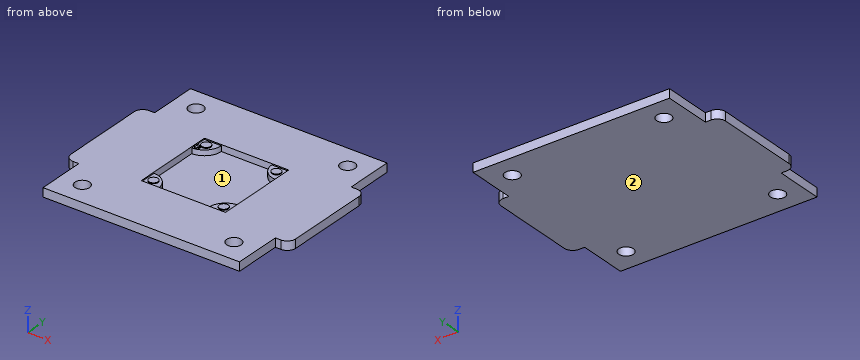
from build123d import *

# Parameters (mm, degrees)
SKETCH_1_W          = 70
SKETCH_1_H          = 70
EXTRUDE_1_DEPTH     = 3.1
SKETCH_2_W          = 30
SKETCH_2_H          = 30
CUT_EXTRUDE_1_DEPTH = 2.3
SKETCH_3_R          = 2.6
CUT_EXTRUDE_2_DEPTH = 4.1
EXTRUDE_2_DEPTH     = 2.7
SKETCH_6_R          = 1.6
EXTRUDE_3_DEPTH     = 0.3


with BuildPart() as part:
    # 草图1 → 凸台-拉伸1 (new body)
    with BuildSketch(Plane.XY):
        with BuildLine():
            Line((-2, 17), (0, 17))
            Line((0, 17), (0, 53))
            Line((0, 53), (-2, 53))
            ThreePointArc((-2, 53), (-4.121320344, 52.121320344), (-5, 50))
            Line((-5, 50), (-5, 20))
            ThreePointArc((-5, 20), (-4.121320344, 17.878679656), (-2, 17))
        make_face()
        with Locations((35, 35)):
            Rectangle(SKETCH_1_W, SKETCH_1_H)
        with BuildLine():
            Line((70, 53), (70, 17))
            Line((70, 17), (72, 17))
            ThreePointArc((72, 17), (74.121320344, 17.878679656), (75, 20))
            Line((75, 20), (75, 50))
            ThreePointArc((75, 50), (74.121320344, 52.121320344), (72, 53))
            Line((72, 53), (70, 53))
        make_face()
    extrude(amount=EXTRUDE_1_DEPTH)

    # 草图2 → 切除-拉伸1 (cut)
    with BuildSketch(Plane.XY.offset(3.1)):
        with Locations((35, 35)):
            Rectangle(SKETCH_2_W, SKETCH_2_H)
    extrude(amount=-CUT_EXTRUDE_1_DEPTH, mode=Mode.SUBTRACT)

    # 草图3 → 切除-拉伸2 (cut, through all)
    with BuildSketch(Plane.XY.offset(3.1)):
        with Locations((8, 62)):
            Circle(SKETCH_3_R)
        with Locations((62, 62)):
            Circle(SKETCH_3_R)
        with Locations((8, 8)):
            Circle(SKETCH_3_R)
        with Locations((62, 8)):
            Circle(SKETCH_3_R)
    extrude(amount=-CUT_EXTRUDE_2_DEPTH, mode=Mode.SUBTRACT)

    # 草图4 → 凸台-拉伸2 (add)
    with BuildSketch(Plane.XY):
        with BuildLine():
            Line((20, 44), (20, 50))
            Line((20, 50), (26, 50))
            ThreePointArc((26, 50), (24.242640687, 45.757359313), (20, 44))
        make_face()
        with BuildLine():
            Line((50, 44), (50, 50))
            Line((50, 50), (44, 50))
            ThreePointArc((44, 50), (45.757359313, 45.757359313), (50, 44))
        make_face()
        with BuildLine():
            Line((50, 20), (44, 20))
            ThreePointArc((44, 20), (45.757359313, 24.242640687), (50, 26))
            Line((50, 26), (50, 20))
        make_face()
        with BuildLine():
            Line((20, 26), (20, 20))
            Line((20, 20), (26, 20))
            ThreePointArc((26, 20), (24.242640687, 24.242640687), (20, 26))
        make_face()
    extrude(amount=EXTRUDE_2_DEPTH)

    # 草图6 → 凸台-拉伸3 (add)
    with BuildSketch(Plane.XY.offset(2.7)):
        with Locations((22.5, 47.5)):
            Circle(SKETCH_6_R)
        with Locations((47.5, 47.5)):
            Circle(SKETCH_6_R)
        with Locations((47.5, 22.5)):
            Circle(SKETCH_6_R)
        with Locations((22.5, 22.5)):
            Circle(SKETCH_6_R)
        Polygon((20.1, 45.5), (20.7, 45.5), (20.7, 46.1), (21.3, 46.1), (21.3, 45.5), (21.9, 45.5), (21.9, 44.9), (21.3, 44.9), (21.3, 44.3), (20.7, 44.3), (20.7, 44.9), (20.1, 44.9), align=None)
    extrude(amount=EXTRUDE_3_DEPTH)


solid = part.part
Geometry check sheet. Reference: the model listing, model coordinates, mm. Face numbers are marked on the shaded views. Round coordinates to 2 decimals unless told otherwise and drop trailing zeros. Loops run counter-clockwise (first coordinate to the right, second up) from the corner with the lowest first, then second, coordinate; pieces in that order, holes last. Notation, with made-up numbers: (-1.5, 41.5) - (34.5, 41.5) arc R26 cw to (34.5, 67.5) - close; hole circle Ø9 at (17.25, 84). An arc over 180 degrees is marked (long way). Answer as CSV lines item,"result".
(1) Cross-section at B-B, the plane z = 1.8. Enter the section's corners in (x, y).
Output values:
outline,"(-5, 20) arc R3 ccw to (-2, 17) - (0, 17) - (0, 0) - (70, 0) - (70, 17) - (72, 17) arc R3 ccw to (75, 20) - (75, 50) arc R3 ccw to (72, 53) - (70, 53) - (70, 70) - (0, 70) - (0, 53) - (-2, 53) arc R3 ccw to (-5, 50) - close; hole circle Ø5.2 at (8, 8); hole circle Ø5.2 at (8, 62); hole (20, 26) arc R6 cw to (26, 20) - (44, 20) arc R6 cw to (50, 26) - (50, 44) arc R6 cw to (44, 50) - (26, 50) arc R6 cw to (20, 44) - close; hole circle Ø5.2 at (62, 8); hole circle Ø5.2 at (62, 62)"
(2) Release check for a two-part mould opening along Y. For the marked faces 1 and 2 record: released by +Y, released by -Y, zero draft, split by the parting line, or undercut.
Output values:
face 1,"undercut"
face 2,"zero draft"
(3) Cross-section at A-A, the plane y = 9. Enter the section's corners in (x, z).
Output values:
outline,"(0, 0) - (5.6, 0) - (5.6, 3.1) - (0, 3.1) - close; (10.4, 0) - (59.6, 0) - (59.6, 3.1) - (10.4, 3.1) - close; (64.4, 0) - (70, 0) - (70, 3.1) - (64.4, 3.1) - close"
(4) Depth check by flat-ended pin: pin 1 Ø1.6 at (x, y) = (47, 47.5) entering from +Z; pin 2 Ø1.6 at (y, z) = (61, 1) entering from +X; pin 3 Ø4.5 at (x, y) = (62, 62) entering from -Z. Enter the tip coordinate at first touch or a pass-through.
Output values:
pin 1,"stops at z = 3"
pin 2,"stops at x = 70"
pin 3,"passes through"
(5) Material ranges on line 1 along Y through (x, z) = (8, 2.25); line 2 along X through (y, z) = (27.5, 1.1); line 3 along Y through (x, z) = (9.5, 0.4), recorded low to high.
Output values:
line 1,"y = 0 to 5.4, 10.6 to 59.4, 64.6 to 70"
line 2,"x = -5 to 20, 50 to 75"
line 3,"y = 0 to 5.88, 10.12 to 59.88, 64.12 to 70"
(6) Cross-section at D-D, the plane y = 36. Enter the section's corners in (x, z).
Output values:
outline,"(-5, 0) - (75, 0) - (75, 3.1) - (50, 3.1) - (50, 0.8) - (20, 0.8) - (20, 3.1) - (-5, 3.1) - close"
(7) Cross-section at C-C, the plane x = 62. Enter the section's corners in (y, z), and give its area (3 significant figures).
Output values:
outline,"(0, 0) - (5.4, 0) - (5.4, 3.1) - (0, 3.1) - close; (10.6, 0) - (59.4, 0) - (59.4, 3.1) - (10.6, 3.1) - close; (64.6, 0) - (70, 0) - (70, 3.1) - (64.6, 3.1) - close"
area,"185 mm²"
